Model file for the job. Use its own axes, mm. Face numbers are marked on the shaded views. A direction names the side the tool comes from. Round coordinates to 2 decimals unless told otherwise and drop trailing zeros. Loops run counter-clockwise (first coordinate to the right, second up) from the corner with the lowest first, then second, coordinate; pieces in that order, holes last. Notation, with made-up numbers: M -27.75,63.5 L -23.75,63.5 A21 ccw -23.75,83.5 Z; hole C -4,13.5 d7. An arc over 180 degrees is marked long. Answer in a Markdown table with one row per item.
from build123d import *

# Parameters (mm, degrees)
SKETCH1_W           = 15
SKETCH1_H           = 40
BOSS_EXTRUDE1_DEPTH = 23
SKETCH2_OUTSIDE_W   = 34.704
SKETCH2_OUTSIDE_H   = 51.704
CUT_EXTRUDE1_DEPTH  = 207.508357771
SKETCH3_R           = 5
CUT_EXTRUDE2_DEPTH  = 207.508357771
SKETCH4_R           = 1.75
CUT_EXTRUDE3_DEPTH  = 17


with BuildPart() as part:
    # Sketch1 → Boss-Extrude1 (new body)
    with BuildSketch(Plane.XY):
        with Locations((243.381155173, -184.674624292)):
            Rectangle(SKETCH1_W, SKETCH1_H)
    extrude(amount=BOSS_EXTRUDE1_DEPTH)

    # Sketch2 outside → Cut-Extrude1 (cut, through all)
    with BuildSketch(Plane(origin=(250.881155173, 0, 0), x_dir=(0, 0, -1), z_dir=(1, 0, 0))):
        with Locations((-11.5, -184.675)):
            Rectangle(SKETCH2_OUTSIDE_W, SKETCH2_OUTSIDE_H)
        with BuildLine():
            Line((-11.5, -173.174624292), (-5.75, -173.174624292))
            Line((-5.75, -173.174624292), (-5.75, -164.674624292))
            Line((-5.75, -164.674624292), (0, -164.674624292))
            Line((0, -164.674624292), (0, -204.674624292))
            Line((0, -204.674624292), (-5.75, -204.674624292))
            Line((-5.75, -204.674624292), (-5.75, -196.174624292))
            Line((-5.75, -196.174624292), (-11.5, -196.174624292))
            ThreePointArc((-11.5, -196.174624292), (-23, -184.674624292), (-11.5, -173.174624292))
        make_face(mode=Mode.SUBTRACT)
    extrude(amount=-CUT_EXTRUDE1_DEPTH, mode=Mode.SUBTRACT)

    # Sketch3 → Cut-Extrude2 (cut, through all)
    with BuildSketch(Plane(origin=(250.881155173, 0, 0), x_dir=(0, 0, -1), z_dir=(1, 0, 0))):
        with Locations((-11.5, -184.674624292)):
            Circle(SKETCH3_R)
    extrude(amount=-CUT_EXTRUDE2_DEPTH, mode=Mode.SUBTRACT)

    # Sketch4 → Cut-Extrude3 (cut)
    with BuildSketch(Plane.XY.offset(5.75)):
        with Locations((243.381155173, -200.424624292)):
            Circle(SKETCH4_R)
        with Locations((243.381155173, -168.924624292)):
            Circle(SKETCH4_R)
    extrude(amount=-CUT_EXTRUDE3_DEPTH, mode=Mode.SUBTRACT)


solid = part.part
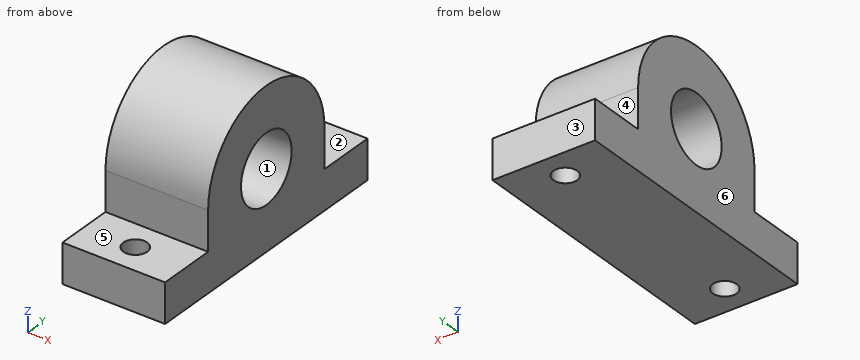
1. Saw through at C-C (z = 9.25). Write the cut outline in (x, y).
Verdict:
| item | result |
|---|---|
| outline | M 235.88,-196.17 L 250.88,-196.17 L 250.88,-189.14 L 235.88,-189.14 Z; M 235.88,-180.21 L 250.88,-180.21 L 250.88,-173.17 L 235.88,-173.17 Z |
2. Mould opens along Y. For the marked faces 1, 2 and 3 say: +Y half, -Y half, draft (parallel to the pull), parting line (faces both ways), or undercut.
Verdict:
| item | result |
|---|---|
| face 1 | undercut |
| face 2 | draft |
| face 3 | +Y half |
3. Tool access for the marked faces 4, 5 and 6: list every direction of +Z, -Z, +X, -X, +Y, -Y with a clear straight run to the whole face (end or side of a thin tool).
Verdict:
| item | result |
|---|---|
| face 4 | +Z, +X, -X, +Y |
| face 5 | +Z, +X, -X, -Y |
| face 6 | +Z, -Z, -X, +Y, -Y |
4. Saw through at A-A (y = -186.5). Write the cut outline in (x, z), and give its area (3 significant figures).
Verdict:
| item | result |
|---|---|
| outline | M 235.88,0 L 250.88,0 L 250.88,6.85 L 235.88,6.85 Z; M 235.88,16.15 L 250.88,16.15 L 250.88,22.85 L 235.88,22.85 Z |
| area | 203 mm² |
5. Pin check, flat tips, straight feed: pin 1 (2 mm diameter, centred on x = 243.38, y = -168.92, fed in from -Z); pin 2 (4 mm diameter, centred on x = 243.5, y = -198.5, fed in from +Z); pin 3 (6 mm diameter, centred on x = 237.5, z = 10, fed in from +Y); pin 4 (6 mm diameter, centred on x = 238, z = 13.5, fed in from -Y). Stop position of each tip, or through.
Verdict:
| item | result |
|---|---|
| pin 1 | passes through |
| pin 2 | stops at z = 5.75 |
| pin 3 | stops at y = -173.17 |
| pin 4 | stops at y = -196.17 |
6. Saw through at B-B (x = 242.5). Write the cut outline in (y, z).
Verdict:
| item | result |
|---|---|
| outline | M -204.67,0 L -201.94,0 L -201.94,5.75 L -204.67,5.75 Z; M -198.91,0 L -170.44,0 L -170.44,5.75 L -173.17,5.75 L -173.17,11.5 A11.5 ccw -196.17,11.5 L -196.17,5.75 L -198.91,5.75 Z; M -167.41,0 L -164.67,0 L -164.67,5.75 L -167.41,5.75 Z; hole C -184.67,11.5 d10 |
7. Saw through at D-D (x = 240.75). Write the cut outline in (y, z), and give its area (3 significant figures).
Verdict:
| item | result |
|---|---|
| outline | M -204.67,0 L -164.67,0 L -164.67,5.75 L -173.17,5.75 L -173.17,11.5 A11.5 ccw -196.17,11.5 L -196.17,5.75 L -204.67,5.75 Z; hole C -184.67,11.5 d10 |
| area | 491 mm² |
8. Wall check: probe 1 along Z at (x, y) = (242.75, -184.5); probe 2 along Y at (x, z) = (246.25, 11.5); probe 3 along Z at (x, y) = (240, -166.5). Give the ranges that are in metal, low to high.
Verdict:
| item | result |
|---|---|
| probe 1 | z = 0 to 6.5, 16.5 to 23 |
| probe 2 | y = -196.17 to -189.67, -179.67 to -173.17 |
| probe 3 | z = 0 to 5.75 |
